Could you check a few things on this model? Use its own coordinates, in mm. Face numbers are marked on the shaded views. A direction names the side the tool comes from. Give positions to 0.01 mm unless a question says otherwise; leave off trailing zeros. Order: outer loops, then holes, each group sorted by start corner. A loop starts at its lowest first (then second) coordinate and runs counter-clockwise, first axis right, second up. Notation, with made-up numbers: (-36.75, -16) - (5.25, -16) arc R22 cw to (5.25, 17) - close; hole circle Ø1 at (75.5, -37). An arc over 180 degrees is marked (long way). Put each result on its own line as item: value.
from build123d import *

# Parameters (mm, degrees)
EXTRUDE_1_OUTLINE_R   = 35
EXTRUDE_1_OUTLINE_R_2 = 1.55
EXTRUDE_1_OUTLINE_R_3 = 30.05
EXTRUDE_1_DEPTH       = 10
SKETCH_2_R            = 33.525
SKETCH_2_R_2          = 18.525
EXTRUDE_1_2_DEPTH     = 4
SKETCH_3_R            = 1.55
CUT_EXTRUDE_1_DEPTH   = 51.497524692
CUT_EXTRUDE_2_DEPTH   = 5


# Read off the part's stored shape, not the designer's step: 凸台-拉伸1
with BuildPart() as part:
    # Extrude 1 outline → Extrude 1 (new body)
    with BuildSketch(Plane.XY):
        Circle(EXTRUDE_1_OUTLINE_R)
        with Locations((0, -32.5)):
            Circle(EXTRUDE_1_OUTLINE_R_2, mode=Mode.SUBTRACT)
        with Locations((-32.5, 0)):
            Circle(EXTRUDE_1_OUTLINE_R_2, mode=Mode.SUBTRACT)
        Circle(EXTRUDE_1_OUTLINE_R_3, mode=Mode.SUBTRACT)
        with Locations((32.5, 0)):
            Circle(EXTRUDE_1_OUTLINE_R_2, mode=Mode.SUBTRACT)
        with Locations((0, 32.5)):
            Circle(EXTRUDE_1_OUTLINE_R_2, mode=Mode.SUBTRACT)
    extrude(amount=EXTRUDE_1_DEPTH)

    # 草图2 → Extrude 1 2 (add)
    with BuildSketch(Plane.XY.offset(10)):
        Circle(SKETCH_2_R)
        Circle(SKETCH_2_R_2, mode=Mode.SUBTRACT)
    extrude(amount=-EXTRUDE_1_2_DEPTH)

    # 草图3 → 切除-拉伸1 (cut, through all)
    with BuildSketch(Plane(origin=(0, 0, 0), x_dir=(-1, 0, 0), z_dir=(0, 0, -1))):
        with Locations(Location((32.5, 0, 0), (0, 0, 180))):
            Circle(SKETCH_3_R)
        with Locations(Location((0, -32.5, 0), (0, 0, 180))):
            Circle(SKETCH_3_R)
        with Locations(Location((-32.5, 0, 0), (0, 0, 180))):
            Circle(SKETCH_3_R)
        with Locations(Location((0, 32.5, 0), (0, 0, 180))):
            Circle(SKETCH_3_R)
    extrude(amount=-CUT_EXTRUDE_1_DEPTH, mode=Mode.SUBTRACT)

    # 草图7 → 切除-拉伸2 (cut)
    with BuildSketch(Plane(origin=(0, 0, 0), x_dir=(-1, 0, 0), z_dir=(0, 0, -1))):
        with BuildLine():
            Line((15.025, 26.024063384), (17.5, 30.310889132))
            ThreePointArc((17.5, 30.310889132), (24.748737342, 24.748737342), (30.310889132, 17.5))
            Line((30.310889132, 17.5), (26.024063384, 15.025))
            ThreePointArc((26.024063384, 15.025), (21.248558775, 21.248558775), (15.025, 26.024063384))
        make_face()
    extrude(amount=-CUT_EXTRUDE_2_DEPTH, mode=Mode.SUBTRACT)


solid = part.part
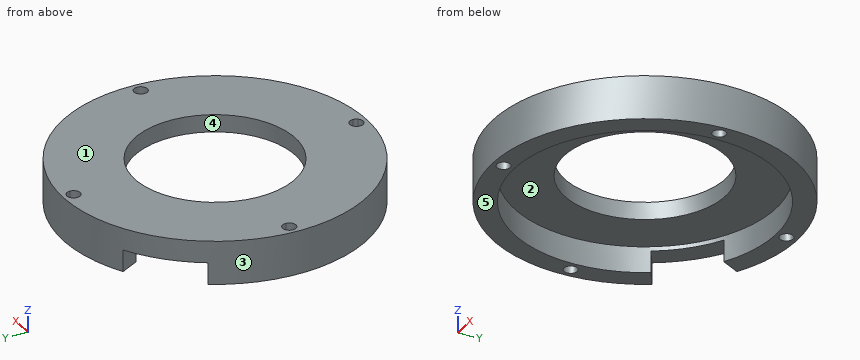
1) We'd pull the mould along X, two halves only. Please class the marked faces 3, 4 and 5: pulls with the +X half, pulls with the -X half, needs draft (parallel to the pull), parting line crosses it, or undercut.
Filled in:
face 3: parting line crosses it
face 4: undercut
face 5: needs draft
2) Suppose I cut it at B-B, the plane z = 1.5. List the corners of the cut face in (x, y) for me (3 decimals).
Filled in:
outline: (-30.311, 17.5) arc R35 ccw (long way) to (-17.5, 30.311) - (-15.025, 26.024) arc R30.05 cw (long way) to (-26.024, 15.025) - close; hole circle Ø3.1 at (-32.5, 0); hole circle Ø3.1 at (0, -32.5); hole circle Ø3.1 at (0, 32.5); hole circle Ø3.1 at (32.5, 0)
3) Suppose I cut it at C-C, the plane y = 8. List the corners of the cut face in (x, z) for me, and give its area (3 significant figures).
Filled in:
outline: (-34.07, 0) - (-28.97, 0) - (-28.97, 6) - (-16.71, 6) - (-16.71, 10) - (-34.07, 10) - close; (16.71, 6) - (28.97, 6) - (28.97, 0) - (34.07, 0) - (34.07, 10) - (16.71, 10) - close
area: 200 mm^2
4) Which directions (+Z, -Z, +X, -X, +Y, -Y) give clear straight access to the entire face, cutting with the end or side of a thin tool? Please do the marked faces 1 and 2.
Filled in:
face 1: +Z, +X, -X, +Y, -Y
face 2: -Z
5) Suppose I cut it at D-D, the plane x = -11.5. List the corners of the cut face in (y, z) for me, and give its area (3 significant figures).
Filled in:
outline: (-33.06, 0) - (-27.76, 0) - (-27.76, 6) - (-14.52, 6) - (-14.52, 10) - (-33.06, 10) - close; (14.52, 6) - (27.76, 6) - (27.76, 0) - (33.06, 0) - (33.06, 10) - (14.52, 10) - close
area: 212 mm^2
6) I'm going to push flat-ended pins straight in: pin 1 (4.5 mm diameter, centred on x = -21.5, y = 22.5, fed in from -Z); pin 2 (6 mm diameter, centred on y = 18, z = 5, fed in from -X); pin 3 (1.5 mm diameter, centred on x = -12, z = 1, fed in from +Y). Where does each tip first touch, or does it pass through?
Filled in:
pin 1: stops at z = 5
pin 2: stops at x = -31.62
pin 3: stops at y = 33.14
7) If I drill on line 1 (Y direction, x = 0, z = 9.15) (3 decimals); line 2 (Y direction, x = 0, z = 2.85); line 3 (Z direction, x = 29, y = 5.5), over which ranges is the centre line in solid material (lowest first)? Write a range as [from, to].
Filled in:
line 1: y = [-35, -34.05], [-30.95, -18.525], [18.525, 30.95], [34.05, 35]
line 2: y = [-35, -34.05], [-30.95, -30.05], [30.05, 30.95], [34.05, 35]
line 3: z = [6, 10]
8) Suppose I cut it at A-A, the plane x = 0. List the corners of the cut face in (y, z) for me (3 decimals), and give its area (3 significant figures).
Filled in:
outline: (-35, 0) - (-34.05, 0) - (-34.05, 10) - (-35, 10) - close; (-30.95, 0) - (-30.05, 0) - (-30.05, 6) - (-18.525, 6) - (-18.525, 10) - (-30.95, 10) - close; (18.525, 6) - (30.05, 6) - (30.05, 0) - (30.95, 0) - (30.95, 10) - (18.525, 10) - close; (34.05, 0) - (35, 0) - (35, 10) - (34.05, 10) - close
area: 129 mm^2
